```python
from build123d import *

# Parameters (mm, degrees)
SKETCH1_R           = 16
SKETCH1_R_2         = 14.35
BOSS_EXTRUDE1_DEPTH = 25
BOSS_EXTRUDE3_DEPTH = 25
BOSS_EXTRUDE4_DEPTH = 16


with BuildPart() as part:
    # Sketch1 → Boss-Extrude1 (new body)
    with BuildSketch(Plane.XY):
        Circle(SKETCH1_R)
        Circle(SKETCH1_R_2, mode=Mode.SUBTRACT)
    extrude(amount=BOSS_EXTRUDE1_DEPTH)

    # Sketch3 → Boss-Extrude3 (add)
    with BuildSketch(Plane.XY):
        with BuildLine():
            Line((16, 16), (0, 16))
            ThreePointArc((0, 16), (11.313708499, 11.313708499), (16, 0))
            Line((16, 0), (16, 16))
        make_face()
        with BuildLine():
            Line((16, -16), (16, 0))
            ThreePointArc((16, 0), (11.313708499, -11.313708499), (0, -16))
            Line((0, -16), (16, -16))
        make_face()
    extrude(amount=BOSS_EXTRUDE3_DEPTH)

    # Sketch2 → Boss-Extrude4 (add)
    with BuildSketch(Plane(origin=(0, 0, 0), x_dir=(0, 0, -1), z_dir=(1, 0, 0))):
        Polygon((-25, 14.35), (-50.4, 39.75), (-50.4, 41.4), (-25, 16), align=None)
        Polygon((-25, -14.35), (-25, -16), (-50.4, -41.4), (-50.4, -39.75), align=None)
    extrude(amount=BOSS_EXTRUDE4_DEPTH)


solid = part.part
```
For this review, take the finished solid that the model builds, in its own axes (mm). A direction names the side the tool comes from. Give positions to 0.01 mm unless a question says otherwise; leave off trailing zeros. Order: outer loops, then holes, each group sorted by start corner. A loop starts at its lowest first (then second) coordinate and runs counter-clockwise, first axis right, second up.
1) Take a section at A-A (z = 41.5). Give the boundary of the cut face in (x, y), then the cut area to 3 significant figures.
2) Take a section at B-B (y = 0). Give the boundary of the cut face in (x, z), then the cut area to 3 significant figures.
3) Take a section at D-D (z = 23.5). Give the boundary of the cut face in (x, y), then the cut area to 3 significant figures.
4) For faces 1 (the face through (7.89, 26.87, 37.52)), 2 (the face through (8, -16, 12)), 3 (the face through (-15, 0, 25)), 4 (the face through (8, 16, 12)), 5 (the face through (14, 4, 0)), list the 3-axis set-ups (+Z, -Z, +X, -X, +Y, -Y) from which the entire face can be reached by the end or side of a thin tool; tool diameter is ignored.
5) Take a section at C-C (x = 12). Give the boundary of the cut face in (y, z).
6) Wall thickness on line 1 (Y direction, x = 0, z = 19); line 2 (X direction, y = -12.5, z = 6.5): over which ranges is each line inside the solid? List them lowest first.
7) Insertion check: pin 1 (8 mm diameter, centred on x = -10.5, y = 4, fed in from +Z); pin 2 (2 mm diameter, centred on x = -10.5, y = 15.5, fed in from -Z); pin 3 (5 mm diameter, centred on x = 3.5, y = -17.5, fed in from +Z); pin 4 (17.5 mm diameter, centred on x = 4, z = 16, fed in from -Y). Each pin has a flat end and moves straight along its axis. Give the tip position at first contact, or say it passes through.
Derived:
1. outline: (0, -32.5) - (16, -32.5) - (16, -30.85) - (0, -30.85) - close; (0, 30.85) - (16, 30.85) - (16, 32.5) - (0, 32.5) - close
1. area: 52.8 mm2
2. outline: (-16, 0) - (-14.35, 0) - (-14.35, 25) - (-16, 25) - close; (14.35, 0) - (16, 0) - (16, 25) - (14.35, 25) - close
2. area: 82.5 mm2
3. outline: (0, -16) - (16, -16) - (16, 16) - (0, 16) arc R16 ccw to start; hole circle Ø28.7 at (0, 0)
3. area: 267 mm2
4. face 1: +Z, +X, -X
4. face 2: -Z, +X, -X, -Y
4. face 3: +Z, -X, +Y, -Y
4. face 4: -Z, +X, -X, +Y
4. face 5: -Z, +X, -X, +Y, -Y
5. outline: (-41.4, 50.4) - (-16, 25) - (-16, 0) - (-7.87, 0) - (-7.87, 25) - (-14.35, 25) - (-39.75, 50.4) - close; (7.87, 0) - (16, 0) - (16, 25) - (41.4, 50.4) - (39.75, 50.4) - (14.35, 25) - (7.87, 25) - close
6. line 1: y = -16 to -14.35, 14.35 to 16
6. line 2: x = -9.99 to -7.05, 7.05 to 16
7. pin 1: stops at z = 25
7. pin 2: passes through
7. pin 3: stops at z = 30.65
7. pin 4: stops at y = -16
